The listing builds one solid part. Answer for the finished solid, in the listing's coordinates (mm). Coordinates: 2 decimals unless noted, no trailing zeros. Loops run counter-clockwise (first coordinate to the right, second up) from the corner with the lowest first, then second, coordinate; pieces in that order, holes last. Notation, with made-up numbers: (-24.5, 15) - (-9.5, 15) arc R20 cw to (-9.5, 37) - close; hole circle Ø4 at (27.25, 54). An arc over 180 degrees is marked (long way). Put each result on its own line as item: value.
```python
from build123d import *

# Parameters (mm, degrees)
SKETCH1_R                      = 100
BOSS_EXTRUDE1_DEPTH            = 7.5
CBORE_FOR_M3_SHCS1_D           = 3.4
CBORE_FOR_M3_SHCS1_DEPTH       = 7.5
CBORE_FOR_M3_SHCS1_CBORE_D     = 6.5
CBORE_FOR_M3_SHCS1_CBORE_DEPTH = 3
CBORE_FOR_M3_SHCS1_TIP         = 1.021463052
CBORE_FOR_M3_SHCS2_D           = 3.6
CBORE_FOR_M3_SHCS2_DEPTH       = 7.5
CBORE_FOR_M3_SHCS2_CBORE_D     = 6.5
CBORE_FOR_M3_SHCS2_CBORE_DEPTH = 3
CBORE_FOR_M3_SHCS2_TIP         = 1.081549114
SKETCH9_W                      = 276.839915284
SKETCH9_H                      = 86.454597136
CUT_EXTRUDE1_DEPTH             = 142.620090383
SKETCH10_R                     = 1.875
CUT_EXTRUDE2_DEPTH             = 1.875
FILLET1_R                      = 1.875


with BuildPart() as part:
    # Sketch1 → Boss-Extrude1 (new body)
    with BuildSketch(Plane(origin=(0, 0, 0), x_dir=(1, 0, 0), z_dir=(0, 1, 0))):
        with Locations(Location((0, 0, 0), (0, 0, 270))):
            Circle(SKETCH1_R)
    extrude(amount=BOSS_EXTRUDE1_DEPTH)

    # CBORE for M3 SHCS1
    with Locations(Plane(origin=(0, 0, 0), x_dir=(-1, 0, 0), z_dir=(0, -1, 0))):
        with Locations((0, -92.5), (-65.40737726, -65.40737726), (-92.5, 0), (-65.40737726, 65.40737726), (0, 92.5), (65.40737726, 65.40737726), (92.5, 0), (65.40737726, -65.40737726)):
            CounterBoreHole(CBORE_FOR_M3_SHCS1_D / 2, CBORE_FOR_M3_SHCS1_CBORE_D / 2, CBORE_FOR_M3_SHCS1_CBORE_DEPTH, depth=CBORE_FOR_M3_SHCS1_DEPTH)
            with Locations((0, 0, -(CBORE_FOR_M3_SHCS1_DEPTH + CBORE_FOR_M3_SHCS1_TIP / 2))):  # 118° drill point
                Cone(0, CBORE_FOR_M3_SHCS1_D / 2, CBORE_FOR_M3_SHCS1_TIP, mode=Mode.SUBTRACT)

    # CBORE for M3 SHCS2
    with Locations(Plane(origin=(0, 0, 0), x_dir=(-1, 0, 0), z_dir=(0, -1, 0))):
        with Locations((-53, 34), (53, 34), (53, -34), (-53, -34)):
            CounterBoreHole(CBORE_FOR_M3_SHCS2_D / 2, CBORE_FOR_M3_SHCS2_CBORE_D / 2, CBORE_FOR_M3_SHCS2_CBORE_DEPTH, depth=CBORE_FOR_M3_SHCS2_DEPTH)
            with Locations((0, 0, -(CBORE_FOR_M3_SHCS2_DEPTH + CBORE_FOR_M3_SHCS2_TIP / 2))):  # 118° drill point
                Cone(0, CBORE_FOR_M3_SHCS2_D / 2, CBORE_FOR_M3_SHCS2_TIP, mode=Mode.SUBTRACT)

    # Sketch9 → Cut-Extrude1 (cut, through all)
    with BuildSketch(Plane(origin=(0, 0, 0), x_dir=(0.3646980843717534, 0, 0.9311258278318637), z_dir=(-0.9311258278318637, 0, 0.3646980843717534))):
        with Locations((-1.022117504, -7.168579764)):
            Rectangle(SKETCH9_W, SKETCH9_H)
    extrude(amount=-CUT_EXTRUDE1_DEPTH, mode=Mode.SUBTRACT)

    # Sketch10 → Cut-Extrude2 (cut)
    with BuildSketch(Plane(origin=(0, 0, 0), x_dir=(0.3646980843717534, 0, 0.9311258278318637), z_dir=(-0.9311258278318637, 0, 0.3646980843717534))):
        with Locations(Location((0, 3.75, 0), (0, 0, 180))):
            Circle(SKETCH10_R)
        with Locations(Location((-40, 3.75, 0), (0, 0, 180))):
            Circle(SKETCH10_R)
        with Locations(Location((-80, 3.75, 0), (0, 0, 180))):
            Circle(SKETCH10_R)
        with Locations(Location((80, 3.75, 0), (0, 0, 180))):
            Circle(SKETCH10_R)
        with Locations(Location((40, 3.75, 0), (0, 0, 180))):
            Circle(SKETCH10_R)
    extrude(amount=CUT_EXTRUDE2_DEPTH, mode=Mode.SUBTRACT)

    # Fillet1
    fillet1_edges = [part.edges().sort_by_distance(p)[0] for p in [
        (-1.062052019, 3.75, 2.429669835),
        (-15.649975394, 3.75, -34.815363278),
        (-30.237898769, 3.75, -72.060396391),
        (28.113794731, 3.75, 76.919736062),
        (13.525871356, 3.75, 39.674702949),
    ]]
    fillet(fillet1_edges, radius=FILLET1_R - 0.0001)  # a hair under: the kernel refuses the full size


solid = part.part
```
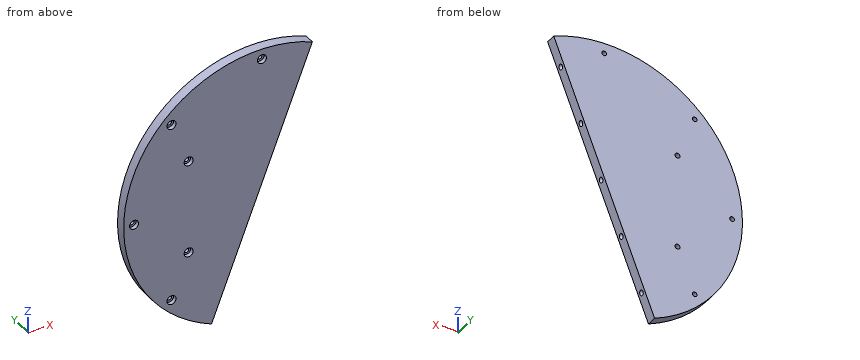
1) Straight lines are drawn through the part: L1, parallel to Z at x = -53, y = 5.35; L2, parallel to X at y = 6.25, z = 92.5; L3, parallel to X at y = 0.5, z = -65. For each, find the intervals that lie inside material, in ascending order. Write a range as [from, to].
Found:
L1: z = [-84.8, -35.8], [-32.2, 32.2], [35.8, 84.8]
L2: x = [-38, -1.7], [1.7, 36.23]
L3: x = [-75.99, -68.63], [-62.18, -25.46]
2) Each of these flat-tipped pins is pushed along its axis until it touches: pin 1 (5 mm diameter, centred on x = -93.5, z = -1, fed in from -Y); pin 2 (4 mm diameter, centred on y = 6, z = 52.5, fed in from -X); pin 3 (1 mm diameter, centred on x = -80, y = 3.5, fed in from +Z); pin 4 (4 mm diameter, centred on x = -53, z = -34, fed in from -Y). Where does it stop, or does it pass through?
Found:
pin 1: stops at y = 0
pin 2: stops at x = -86.31
pin 3: stops at z = 60.66
pin 4: stops at y = 3
3) The part is cut by section A-A (x = -74.5). Give the vertices of the cut face in (y, z).
Found:
outline: (0, -66.71) - (7.5, -66.71) - (7.5, 66.71) - (0, 66.71) - close
